For this review, take the finished solid that the model builds, in its own axes (mm). A direction names the side the tool comes from. Give positions to 0.01 mm unless a question says otherwise; leave off trailing zeros. One line per item, written item: value. Start each with the question number.
Item 1: Tool access review of faces 3 (the face through (-1, -0.125, 0)), 4 (the face through (-33.99, 2.46, -29.24)): name each direction out of +Z, -Z, +X, -X, +Y, -Y from which nothing blocks a thin tool from reaching the whole face with its end or side.
Item 2: To check wall thickness, follow probe 1 along X at (y, z) = (4.05, 0.5); probe 2 along Z at (x, y) = (-2, 4.65); probe 3 along X at (y, z) = (0.8, -8). State the ranges of each line that lie inside material, in increasing order.
Item 3: Mouldability with a two-part tool opening along X and no side actions: class faces 1 (the face through (33.99, 2.46, 29.24)), 2 (the face through (0, 5.125, 1)) as released by +X, released by -X, zero draft, split by the parting line, or undercut.
```python
from build123d import *

# Parameters (mm, degrees)
SKETCH1_W               = 100
SKETCH1_H               = 60
BOSS_EXTRUDE1_DEPTH     = 5
BOSS_EXTRUDE1_TAPER     = 1
FILLET1_R               = 5
SKETCH2_R               = 1.5
CUT_EXTRUDE1_DEPTH      = 5
CUT_EXTRUDE1_TAPER      = -1
MIRROR2_COPY_1_SKETCH_R = 1.5
MIRROR2_COPY_1_DEPTH    = 5
MIRROR2_COPY_1_TAPER    = -1
SCALE1_SCALE            = 1.05


with BuildPart() as part:
    # Sketch1 → Boss-Extrude1 (new body)
    with BuildSketch(Plane(origin=(0, 0, 0), x_dir=(1, 0, 0), z_dir=(0, 1, 0))):
        Rectangle(SKETCH1_W, SKETCH1_H)
    extrude(amount=BOSS_EXTRUDE1_DEPTH, taper=BOSS_EXTRUDE1_TAPER)

    # Fillet1
    fillet1_edges = [part.edges().sort_by_distance(p)[0] for p in [
        (49.956362338, 2.5, 29.956362338),
        (-49.956362338, 2.5, 29.956362338),
        (-49.956362338, 2.5, -29.956362338),
        (49.956362338, 2.5, -29.956362338),
    ]]
    fillet(fillet1_edges, radius=FILLET1_R)

    # Sketch2 → Cut-Extrude1 (cut)
    with BuildSketch(Plane(origin=(0, 5, 0), x_dir=(1, 0, 0), z_dir=(0, 1, 0))):
        with Locations((33.912724675, -27.912724675)):
            Circle(SKETCH2_R)
    cut_extrude1 = extrude(amount=-CUT_EXTRUDE1_DEPTH, taper=CUT_EXTRUDE1_TAPER, mode=Mode.SUBTRACT)

    # Mirror1: Cut-Extrude1 across plane
    add(cut_extrude1.mirror(Plane.XY), mode=Mode.SUBTRACT)

    # Mirror2: Cut-Extrude1 across plane
    add(cut_extrude1.mirror(Plane(origin=(0, 0, 0), x_dir=(0, 0, 1), z_dir=(1, 0, 0))), mode=Mode.SUBTRACT)

    # Mirror2 copy 1 sketch → Mirror2 copy 1 (cut)
    with BuildSketch(Plane(origin=(0, 5, 0), x_dir=(-1, 0, 0), z_dir=(0, 1, 0))):
        with Locations((33.912724675, -27.912724675)):
            Circle(MIRROR2_COPY_1_SKETCH_R)
    extrude(amount=-MIRROR2_COPY_1_DEPTH, taper=MIRROR2_COPY_1_TAPER, mode=Mode.SUBTRACT)


with BuildPart() as part_1:
    # Scale1: scaled about (-4.1e-08, 2.498279052, 6.8e-08)
    add(part.part.scale(SCALE1_SCALE).moved(Location((2e-09, -0.124913953, -3e-09))))


solid = part_1.part
```
Model answer:
1. face 3: +Z, -Z, +X, -X, -Y
1. face 4: -Y
2. probe 1: x = -52.43 to 52.43
2. probe 2: z = -31.42 to 31.42
2. probe 3: x = -52.48 to 52.48
3. face 1: undercut
3. face 2: zero draft
